Read the model definition and answer for the solid it produces. Units are mm, in the model's axes. A direction names the side the tool comes from. Coordinates: 2 decimals unless noted, no trailing zeros. Loops run counter-clockwise (first coordinate to the right, second up) from the corner with the lowest first, then second, coordinate; pieces in that order, holes last. Notation, with made-up numbers: (-15.75, 77.25) - (-1.75, 77.25) arc R21 cw to (-1.75, 116.25) - close; hole circle Ø2 at (60.5, 47). An arc over 180 degrees is marked (long way). Use one line per item in the form item = value.
from build123d import *

# Parameters (mm, degrees)
SKETCH_1_W          = 42.3
SKETCH_1_H          = 42.3
EXTRUDE_1_DEPTH     = 30
CHAMFER_1_SIZE      = 2
SKETCH_2_R          = 1.5
CUT_EXTRUDE_1_DEPTH = 3
SKETCH_3_R          = 11
EXTRUDE_2_DEPTH     = 2
SKETCH_4_R          = 2.5
EXTRUDE_3_DEPTH     = 22


with BuildPart() as part:
    # 草图1 → 凸台-拉伸1 (new body)
    with BuildSketch(Plane(origin=(0, 0, 0), x_dir=(0, 0, -1), z_dir=(1, 0, 0))):
        Rectangle(SKETCH_1_W, SKETCH_1_H)
    extrude(amount=EXTRUDE_1_DEPTH)

    # 倒角1
    chamfer_1_edges = [part.edges().sort_by_distance(p)[0] for p in [
        (15, 21.15, 21.15),
        (15, 21.15, -21.15),
        (15, -21.15, -21.15),
        (15, -21.15, 21.15),
    ]]
    chamfer(chamfer_1_edges, length=CHAMFER_1_SIZE)

    # 草图2 → 切除-拉伸1 (cut)
    with BuildSketch(Plane(origin=(30, 0, 0), x_dir=(0, 0, -1), z_dir=(1, 0, 0))):
        with Locations((-15.5, 15.5)):
            Circle(SKETCH_2_R)
        with Locations((15.5, 15.5)):
            Circle(SKETCH_2_R)
        with Locations((15.5, -15.5)):
            Circle(SKETCH_2_R)
        with Locations((-15.5, -15.5)):
            Circle(SKETCH_2_R)
    extrude(amount=-CUT_EXTRUDE_1_DEPTH, mode=Mode.SUBTRACT)

    # 草图3 → 凸台-拉伸2 (add)
    with BuildSketch(Plane(origin=(30, 0, 0), x_dir=(0, 0, -1), z_dir=(1, 0, 0))):
        Circle(SKETCH_3_R)
    extrude(amount=EXTRUDE_2_DEPTH)

    # 草图4 → 凸台-拉伸3 (add)
    with BuildSketch(Plane(origin=(32, 0, 0), x_dir=(0, 0, -1), z_dir=(1, 0, 0))):
        Circle(SKETCH_4_R)
    extrude(amount=EXTRUDE_3_DEPTH)


solid = part.part
Item 1: The part is cut by section A-A on x = 28. Give the vertices of the cut face in (y, z), plus the area to 3 significant figures.
Results below:
outline = (-21.15, -19.15) - (-19.15, -21.15) - (19.15, -21.15) - (21.15, -19.15) - (21.15, 19.15) - (19.15, 21.15) - (-19.15, 21.15) - (-21.15, 19.15) - close; hole circle Ø3 at (-15.5, -15.5); hole circle Ø3 at (-15.5, 15.5); hole circle Ø3 at (15.5, -15.5); hole circle Ø3 at (15.5, 15.5)
area = 1,750 mm²
Item 2: The part is cut by section B-B on y = 15.5. Give the vertices of the cut face in (x, z).
Results below:
outline = (0, -21.15) - (30, -21.15) - (30, -17) - (27, -17) - (27, -14) - (30, -14) - (30, 14) - (27, 14) - (27, 17) - (30, 17) - (30, 21.15) - (0, 21.15) - close
Item 3: Find the intervals of material crossed by L1, parallel to Y at x = 28.15, z = -15.5; L2, parallel to Y at x = 28, z = 15, in increasing order.
Results below:
L1 = -21.15 to -17, -14 to 14, 17 to 21.15
L2 = -21.15 to -16.91, -14.09 to 14.09, 16.91 to 21.15
Item 4: Which of the six approach directions +Z, -Z, +X, -X, +Y, -Y give full straight-line access (tool end or side, diameter ignored) to faces 5 (the cylindrical face through (28.52, 15.57, -14)), 6 (the flat face through (15, -21.15, 0))?
Results below:
face_5 = +X
face_6 = +Z, -Z, +X, -X, -Y
Item 5: For a pull along Z with two mould halves and no side action, classify faces 1 (the flat face through (27, -15, 16)), 2 (the flat face through (14.8, 20.2, -20.1)), 3 (the cylindrical face through (28.52, -15.43, -14)), 4 (the flat face through (30, -9, 10)) as +Z half, -Z half, draft (parallel to the pull), parting line (faces both ways), or undercut.
Results below:
face_1 = undercut
face_2 = -Z half
face_3 = undercut
face_4 = draft
Item 6: The part is cut by section D-D on x = 41. Give the vertices of the cut face in (y, z), plus the area to 3 significant figures.
Results below:
outline = circle Ø5 at (0, 0)
area = 19.6 mm²
Item 7: The part is cut by section C-C on z = 0. Give the vertices of the cut face in (x, y), plus the area to 3 significant figures.
Results below:
outline = (0, -21.15) - (30, -21.15) - (30, -11) - (32, -11) - (32, -2.5) - (54, -2.5) - (54, 2.5) - (32, 2.5) - (32, 11) - (30, 11) - (30, 21.15) - (0, 21.15) - close
area = 1,420 mm²
Item 8: Each of these flat-tipped pins is pushed along its axis until it touches: P1, Ø0.9, axis at y = -15, z = -15.5, coming from the +X side; P2, Ø2.5, axis at y = 16, z = -15.5, coming from the +X side; P3, Ø10, axis at y = -13, z = 5.5, coming from the +X side; P4, Ø3, axis at x = 35, y = 4.5, coming from the +Z side. Where does it stop, or does it pass through?
Results below:
P1 = 27
P2 = 30
P3 = 32
P4 = through
